Part model, mm, in its own coordinate system. Face numbers are marked on the shaded views. A direction names the side the tool comes from. Give positions to 0.01 mm unless a question says otherwise; leave off trailing zeros. Write each loop counter-clockwise with the first axis right and the second up, starting at its lowest first coordinate (ties: lowest second). Pieces come first, ordered by that corner, then holes.
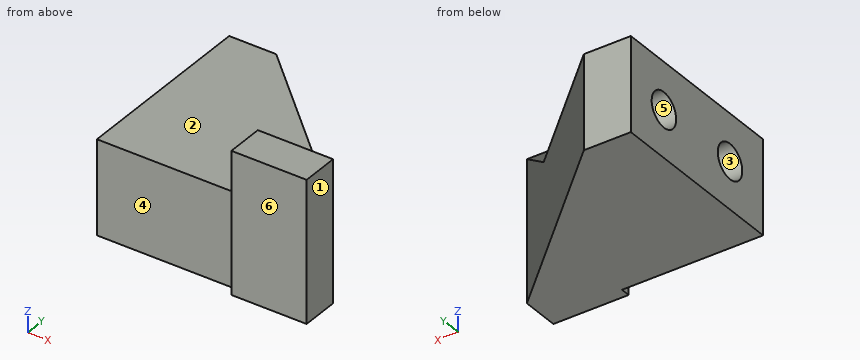
```python
from build123d import *

# Parameters (mm, degrees)
EXTRUDE_1_DEPTH     = 10
SKETCH_2_R          = 1.85
CUT_EXTRUDE_1_DEPTH = 6
SKETCH_3_W          = 8
SKETCH_3_H          = 3
EXTRUDE_2_DEPTH     = 5
CHAMFER_2_SIZE      = 5
SKETCH_4_W          = 8
SKETCH_4_H          = 15
EXTRUDE_3_DEPTH     = 1


with BuildPart() as part:
    # ｽｹｯﾁ1 → ﾎﾞｽ - 押し出し1 (new body)
    with BuildSketch(Plane.XY):
        Polygon((0, 0), (0, 20), (5, 20), (23, 3), (23, 0), align=None)
    extrude(amount=EXTRUDE_1_DEPTH)

    # ｽｹｯﾁ2 → ｶｯﾄ - 押し出し1 (cut)
    with BuildSketch(Plane.ZY):
        with Locations((5, 15)):
            Circle(SKETCH_2_R)
        with Locations((5, 5)):
            Circle(SKETCH_2_R)
    extrude(amount=-CUT_EXTRUDE_1_DEPTH, mode=Mode.SUBTRACT)

    # ｽｹｯﾁ3 → ﾎﾞｽ - 押し出し2 (add)
    with BuildSketch(Plane.XY.offset(10)):
        with Locations((19, 1.5)):
            Rectangle(SKETCH_3_W, SKETCH_3_H)
    extrude(amount=EXTRUDE_2_DEPTH)

    # 面取り2
    chamfer_2_edges = [part.edges().sort_by_distance(p)[0] for p in [
        (19, 3, 10),
    ]]
    chamfer(chamfer_2_edges, length=CHAMFER_2_SIZE - 0.0001)  # a hair under: the kernel refuses the full size

    # ｽｹｯﾁ4 → ﾎﾞｽ - 押し出し3 (add)
    with BuildSketch(Plane(origin=(0, 0, 0), x_dir=(-1, 0, 0), z_dir=(0, -1, 0))):
        with Locations((-19, -7.5)):
            Rectangle(SKETCH_4_W, SKETCH_4_H)
    extrude(amount=EXTRUDE_3_DEPTH)


solid = part.part
```
1) Wall check: L1, parallel to Y at x = 5.25, z = 6.5; L2, parallel to Y at x = 3.65, z = 5; L3, parallel to Z at x = 2.5, y = 1.5. Give the ranges that are in metal, low to high.
Answers follow:
L1: y = 0 to 3.92, 6.08 to 13.92, 16.08 to 19.76
L2: y = 0 to 3.15, 6.85 to 13.15, 16.85 to 20
L3: z = 0 to 10
2) Saw through at B-B, the plane x = 2.5. Write the cut outline in (y, z).
Answers follow:
outline: (0, 0) - (20, 0) - (20, 10) - (0, 10) - close; hole circle Ø3.7 at (5, 5); hole circle Ø3.7 at (15, 5)
3) Pin check, flat tips, straight feed: pin 1 Ø3 at (x, z) = (8.5, 7) entering from -Y; pin 2 Ø9 at (x, y) = (10, 11) entering from +Z; pin 3 Ø12 at (x, y) = (20.5, 15.5) entering from +Z (3 decimals); pin 4 Ø3 at (y, z) = (17.5, 2.5) entering from +X. Stop position of each tip, or through.
Answers follow:
pin 1: stops at y = 0
pin 2: stops at z = 10
pin 3: passes through
pin 4: stops at x = 9.24
4) Saw through at A-A, the plane z = 5. Write the cut outline in (x, y).
Answers follow:
outline: (0, 0) - (15, 0) - (15, -1) - (23, -1) - (23, 3) - (5, 20) - (0, 20) - (0, 16.85) - (6, 16.85) - (6, 13.15) - (0, 13.15) - (0, 6.85) - (6, 6.85) - (6, 3.15) - (0, 3.15) - close
5) Two-plate mould, pull along Z, no slides. Class the marked faces 1, 2 and 3: +Z half, -Z half, draft (parallel to the pull), parting line (faces both ways), or undercut.
Answers follow:
face 1: draft
face 2: +Z half
face 3: undercut
6) 3-axis set-ups, long thin cutter, end or side, ignore diameter. For the marked faces 4, 5 and 6: which of +Z, -Z, +X, -X, +Y, -Y reach the whole face in a straight line?
Answers follow:
face 4: +Z, -Z, -X, -Y
face 5: -X
face 6: +Z, -Z, +X, -X, -Y
7) Saw through at C-C, the plane y = 5. Write the cut outline in (x, z), then the cut area to 3 significant figures.
Answers follow:
outline: (0, 0) - (20.88, 0) - (20.88, 13) - (15, 13) - (15, 10) - (0, 10) - (0, 6.85) - (6, 6.85) - (6, 3.15) - (0, 3.15) - close
area: 204 mm2
